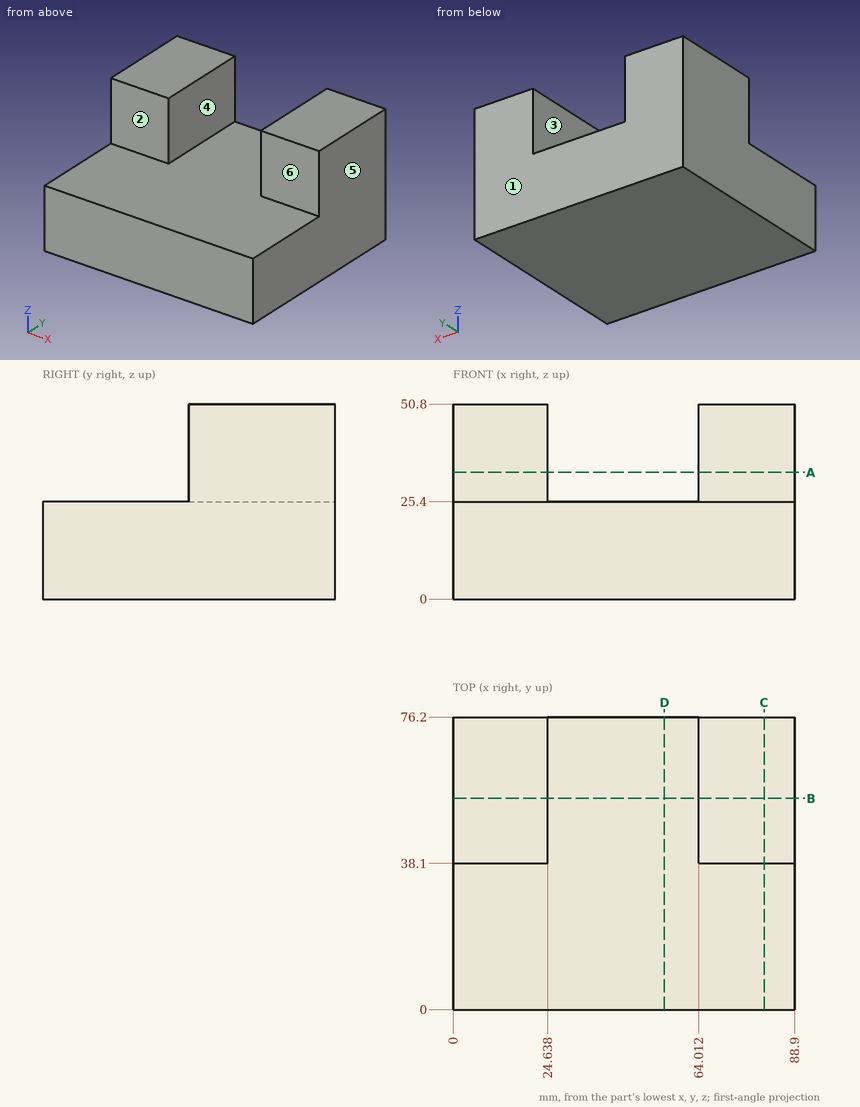
Answer from the drawing. Dimensions are ordinates in mm from the lowest x, y and z of the part. A direction names the side the tool comes from. Give positions to 0.01 mm unless a question says otherwise; leave off trailing zeros. Order: outer loops, then holes, each group sorted by start corner. A loop starts at its lowest first (then second) coordinate and runs counter-clockwise, first axis right, second up. Notation, with made-up numbers: (7.25, 67.5) - (18.25, 67.5) arc R28 cw to (18.25, 106.5) - close; hole circle Ø10 at (75.25, 78). An arc over 180 degrees is marked (long way). Use one line per item in the form item = value.
1) The mould has two halves that part along X. Classify the marked faces 4, 5 and 6: released by +X, released by -X, zero draft, split by the parting line, or undercut.
Verdict:
face_4 = undercut
face_5 = released by +X
face_6 = zero draft
2) Find section D-D on x = 55. Determine the outline of the cut face in (y, z), and give its area (3 significant figures).
Verdict:
outline = (0, 0) - (76.2, 0) - (76.2, 25.4) - (0, 25.4) - close
area = 1,940 mm^2
3) Find section B-B on y = 55. Determine the outline of the cut face in (x, z).
Verdict:
outline = (0, 0) - (88.9, 0) - (88.9, 50.8) - (64.01, 50.8) - (64.01, 25.4) - (24.64, 25.4) - (24.64, 50.8) - (0, 50.8) - close
4) Find section C-C on x = 81. Determine the outline of the cut face in (y, z).
Verdict:
outline = (0, 0) - (76.2, 0) - (76.2, 50.8) - (38.1, 50.8) - (38.1, 25.4) - (0, 25.4) - close
5) Find section A-A on z = 33. Determine the outline of the cut face in (x, y), and give its area (3 significant figures).
Verdict:
outline = (0, 38.1) - (24.64, 38.1) - (24.64, 76.2) - (0, 76.2) - close; (64.01, 38.1) - (88.9, 38.1) - (88.9, 76.2) - (64.01, 76.2) - close
area = 1,890 mm^2
6) This flat-tipped pin is pushed along its axis until it touches: pin 1 (1 mm diameter, centred on x = 21.5, z = 43.5, fed in from -Y). Where does it stop, or does it pass through?
Verdict:
pin_1 = 38.1
7) For the marked faces 1, 2 and 3, determine the directions among +Z, -Z, +X, -X, +Y, -Y from which every point of the face is accessible in a straight line to the end or side of a thin tool.
Verdict:
face_1 = +Z, -Z, +X, -X, +Y
face_2 = +Z, +X, -X, -Y
face_3 = +Z, +Y, -Y
8) Consider probe 1 along X at (y, z) = (72.5, 27); probe 2 along Z at (x, y) = (47, 36); probe 3 along Y at (x, z) = (75, 33). Determine where each line is inside the solid, lowest interval first. Write a range as [from, to].
Verdict:
probe_1 = [0, 24.64], [64.01, 88.9]
probe_2 = [0, 25.4]
probe_3 = [38.1, 76.2]
